from build123d import *

# Parameters (mm, degrees)
SKETCH1_R         = 49
EXTRUDE1_DEPTH    = 85.09
SKETCH5_R         = 3.96875
EXTRUDE5_DEPTH    = 26.67
SKETCH2_OUTSIDE_W = 132.526
SKETCH2_OUTSIDE_H = 132.526
SKETCH2_OUTSIDE_R = 14.2875
EXTRUDE2_DEPTH    = 28.956
SKETCH3_OUTSIDE_W = 132.526
SKETCH3_OUTSIDE_H = 132.526
SKETCH3_OUTSIDE_R = 24.13
EXTRUDE3_DEPTH    = 12.7762
SKETCH4_OUTSIDE_W = 132.526
SKETCH4_OUTSIDE_H = 132.526
SKETCH4_OUTSIDE_R = 46.228
EXTRUDE4_DEPTH    = 32.9057
SKETCH6_R         = 44.45
SKETCH6_R_2       = 24.13
EXTRUDE8_DEPTH    = 23.368
SKETCH7_R         = 19.05
EXTRUDE9_DEPTH    = 50.8
SKETCH8_OUTSIDE_W = 132.526
SKETCH8_OUTSIDE_H = 132.526
SKETCH8_OUTSIDE_R = 41.783
EXTRUDE10_DEPTH   = 7.112


with BuildPart() as part:
    # Sketch1 → Extrude1 (new body)
    with BuildSketch(Plane.XY):
        Circle(SKETCH1_R)
    extrude(amount=EXTRUDE1_DEPTH)

    # Sketch5 → Extrude5 (cut)
    with BuildSketch(Plane.XY.offset(85.09)):
        Circle(SKETCH5_R)
    extrude(amount=-EXTRUDE5_DEPTH, mode=Mode.SUBTRACT)

    # Sketch2 outside → Extrude2 (cut)
    with BuildSketch(Plane.XY.offset(85.09)):
        Rectangle(SKETCH2_OUTSIDE_W, SKETCH2_OUTSIDE_H)
        Circle(SKETCH2_OUTSIDE_R, mode=Mode.SUBTRACT)
    extrude(amount=-EXTRUDE2_DEPTH, mode=Mode.SUBTRACT)

    # Sketch3 outside → Extrude3 (cut)
    with BuildSketch(Plane.XY.offset(56.134)):
        Rectangle(SKETCH3_OUTSIDE_W, SKETCH3_OUTSIDE_H)
        Circle(SKETCH3_OUTSIDE_R, mode=Mode.SUBTRACT)
    extrude(amount=-EXTRUDE3_DEPTH, mode=Mode.SUBTRACT)

    # Sketch4 outside → Extrude4 (cut)
    with BuildSketch(Plane(origin=(0, 0, 0), x_dir=(-1, 0, 0), z_dir=(0, 0, -1))):
        Rectangle(SKETCH4_OUTSIDE_W, SKETCH4_OUTSIDE_H)
        Circle(SKETCH4_OUTSIDE_R, mode=Mode.SUBTRACT)
    extrude(amount=-EXTRUDE4_DEPTH, mode=Mode.SUBTRACT)

    # Sketch6 → Extrude8 (cut)
    with BuildSketch(Plane.XY.offset(43.3578)):
        Circle(SKETCH6_R)
        Circle(SKETCH6_R_2, mode=Mode.SUBTRACT)
    extrude(amount=-EXTRUDE8_DEPTH, mode=Mode.SUBTRACT)

    # Sketch7 → Extrude9 (cut)
    with BuildSketch(Plane(origin=(0, 0, 0), x_dir=(-1, 0, 0), z_dir=(0, 0, -1))):
        Circle(SKETCH7_R)
    extrude(amount=-EXTRUDE9_DEPTH, mode=Mode.SUBTRACT)

    # Sketch8 outside → Extrude10 (cut)
    with BuildSketch(Plane(origin=(0, 0, 0), x_dir=(-1, 0, 0), z_dir=(0, 0, -1))):
        Rectangle(SKETCH8_OUTSIDE_W, SKETCH8_OUTSIDE_H)
        Circle(SKETCH8_OUTSIDE_R, mode=Mode.SUBTRACT)
    extrude(amount=-EXTRUDE10_DEPTH, mode=Mode.SUBTRACT)


solid = part.part
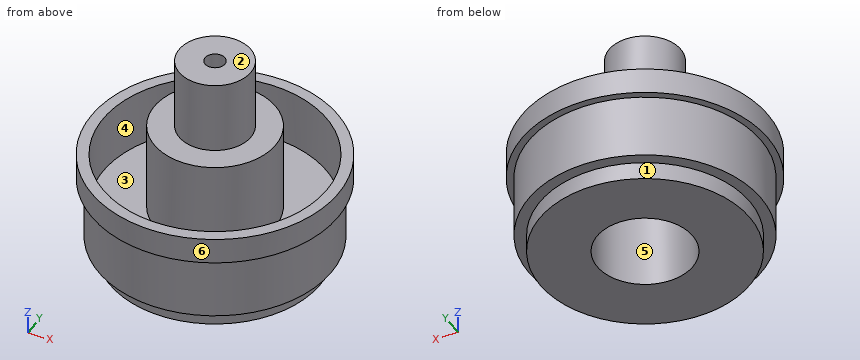
Part model, mm, in its own coordinate system. Face numbers are marked on the shaded views. A direction names the side the tool comes from. Give positions to 0.01 mm unless a question says otherwise; leave off trailing zeros. Order: outer loops, then holes, each group sorted by start corner. A loop starts at its lowest first (then second) coordinate and runs counter-clockwise, first axis right, second up. Notation, with made-up numbers: (-3, -7.5) -> (45, -7.5) arc R16 ccw to (45, -1.5) -> close; hole circle Ø9 at (41.5, -12). An arc over 180 degrees is marked (long way). Use one line per item in the form item = value.
(1) Saw through at C-C (z = 79.5). Write the cut outline in (x, y) (1 decimal).
Solution:
outline = circle Ø28.6 at (0, 0); hole circle Ø7.9 at (0, 0)
(2) Pull direction Y, two halves, no side cores. Call the marked faces 1, 2 and 3: +Y half, -Y half, draft (parallel to the pull), parting line (faces both ways), or undercut.
Solution:
face_1 = parting line
face_2 = draft
face_3 = undercut
(3) Tool access for the marked faces 4, 5 and 6: list every direction of +Z, -Z, +X, -X, +Y, -Y with a clear straight run to the whole face (end or side of a thin tool).
Solution:
face_4 = +Z
face_5 = -Z
face_6 = +Z, -Z
(4) Flat gauge pins, fed straight in: P1, Ø1, axis at x = 11.5, y = -30, coming from the -Z side; P2, Ø2.5, axis at x = 1, y = 0.5, coming from the +Z side; P3, Ø2, axis at x = -29.5, z = 26.5, coming from the -Y side; P4, Ø5, axis at x = 14.5, z = 66, coming from the +Y side. Where does each tip first touch, or does it go through?
Solution:
P1 = 0
P2 = 58.42
P3 = -36.4
P4 = 7.75
(5) Drill centre lines: line 1 (Y direction, x = 0, z = 40.5); line 2 (Y direction, x = 0, z = 26.5); line 3 (Y direction, x = 0, z = 65.5). Where is each one in solid material? Low to high. Write a range as from..to.
Solution:
line_1 = -49..-44.45, -24.13..-19.05, 19.05..24.13, 44.45..49
line_2 = -46.23..-44.45, -24.13..-19.05, 19.05..24.13, 44.45..46.23
line_3 = -14.29..-3.97, 3.97..14.29
(6) Saw through at D-D (y = -16.5). Write the cut outline in (x, z), then the cut area to 3 significant figures.
Solution:
outline = (-46.14, 32.91) -> (-43.18, 32.91) -> (-43.18, 7.11) -> (-38.39, 7.11) -> (-38.39, 0) -> (-9.52, 0) -> (-9.52, 50.8) -> (9.52, 50.8) -> (9.52, 0) -> (38.39, 0) -> (38.39, 7.11) -> (43.18, 7.11) -> (43.18, 32.91) -> (46.14, 32.91) -> (46.14, 43.36) -> (41.27, 43.36) -> (41.27, 19.99) -> (17.61, 19.99) -> (17.61, 56.13) -> (-17.61, 56.13) -> (-17.61, 19.99) -> (-41.27, 19.99) -> (-41.27, 43.36) -> (-46.14, 43.36) -> close
area = 2,110 mm²
